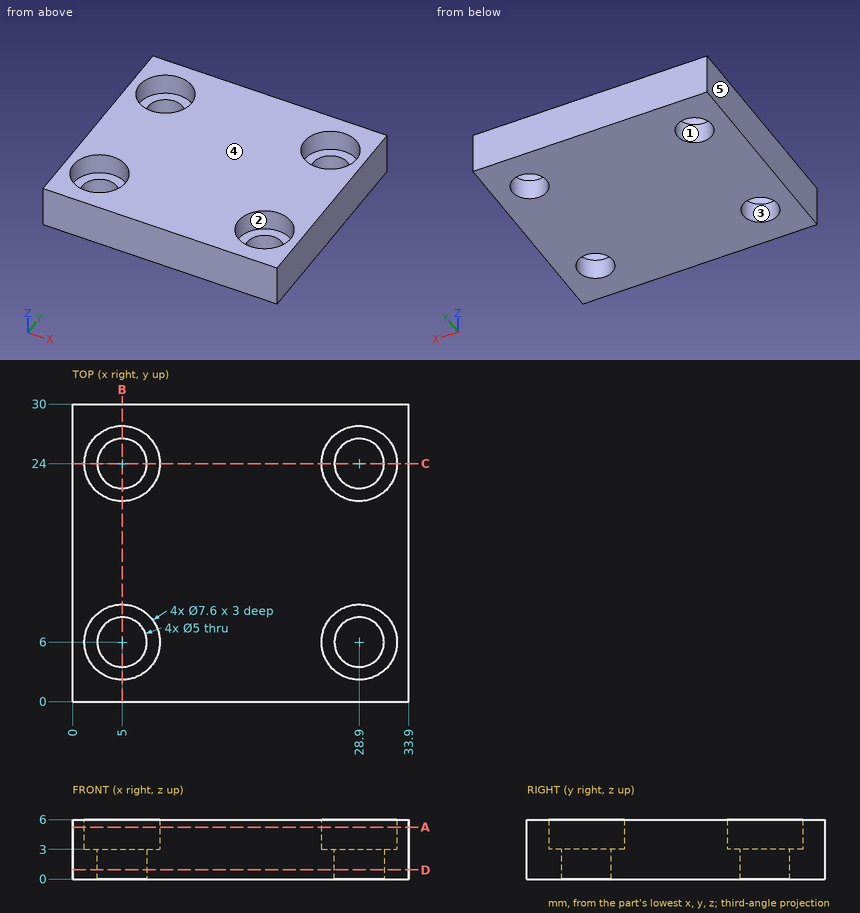
Can you work these out from the drawing? Everything is in mm from the part's minimum corner. A direction names the side the tool comes from. Give positions to 0.01 mm unless a question says otherwise; leave off trailing zeros. Order: outer loops, then holes, each group sorted by start corner. A loop starts at its lowest first (then second) coordinate and runs counter-clockwise, first axis right, second up. Notation, with made-up numbers: M 51.5,44.5 L 58.5,44.5 A24 cw 58.5,81.5 Z; hole C -22,44.25 d5. An arc over 180 degrees is marked long. Write item = value, one per line. Start each with the question number.
Q1. Suppose I cut it at A-A (z = 5.25). Write out the boundary of the cut face in (x, y), plus the area to 3 significant figures.
Q2. Suppose I cut it at C-C (y = 24). Write out the boundary of the cut face in (x, z).
Q3. For the marked faces 1 and 2, which set-ups out of +Z, -Z, +X, -X, +Y, -Y let a thin tool reach every point of the face, with its end or its side?
Q4. Will these pins go through, and if not, where does the flat tip stop? pin 1 Ø7 at (x, y) = (28.9, 6) entering from +Z; pin 2 Ø2 at (y, z) = (12, 1.5) entering from -X; pin 3 Ø2.5 at (x, y) = (6, 6) entering from +Z.
Q5. We'd pull the mould along X, two halves only. Please class the marked faces 3, 4 and 5: pulls with the +X half, pulls with the -X half, needs draft (parallel to the pull), parting line crosses it, or undercut.
Q6. I need wall thicknesses on probe 1 along Y at (x, z) = (28.9, 0.8); probe 2 along Y at (x, z) = (5, 3.3); probe 3 along X at (y, z) = (4.5, 5.15). Which ranges of each line are inside material? Lowest first, please. Write a range as [from, to].
Q7. Suppose I cut it at D-D (z = 0.95). Write out the boundary of the cut face in (x, y), plus the area to 3 significant figures.
Q8. Suppose I cut it at B-B (x = 5). Write out the boundary of the cut face in (y, z).
Check result:
q1.outline = M 0,0 L 33.9,0 L 33.9,30 L 0,30 Z; hole C 5,6 d7.6; hole C 5,24 d7.6; hole C 28.9,6 d7.6; hole C 28.9,24 d7.6
q1.area = 836 mm2
q2.outline = M 0,0 L 2.5,0 L 2.5,3 L 1.2,3 L 1.2,6 L 0,6 Z; M 7.5,0 L 26.4,0 L 26.4,3 L 25.1,3 L 25.1,6 L 8.8,6 L 8.8,3 L 7.5,3 Z; M 31.4,0 L 33.9,0 L 33.9,6 L 32.7,6 L 32.7,3 L 31.4,3 Z
q3.face_1 = +Z, -Z
q3.face_2 = +Z
q4.pin_1 = 3
q4.pin_2 = 0
q4.pin_3 = through
q5.face_3 = undercut
q5.face_4 = needs draft
q5.face_5 = pulls with the -X half
q6.probe_1 = [0, 3.5], [8.5, 21.5], [26.5, 30]
q6.probe_2 = [0, 2.2], [9.8, 20.2], [27.8, 30]
q6.probe_3 = [0, 1.51], [8.49, 25.41], [32.39, 33.9]
q7.outline = M 0,0 L 33.9,0 L 33.9,30 L 0,30 Z; hole C 5,6 d5; hole C 5,24 d5; hole C 28.9,6 d5; hole C 28.9,24 d5
q7.area = 938 mm2
q8.outline = M 0,0 L 3.5,0 L 3.5,3 L 2.2,3 L 2.2,6 L 0,6 Z; M 8.5,0 L 21.5,0 L 21.5,3 L 20.2,3 L 20.2,6 L 9.8,6 L 9.8,3 L 8.5,3 Z; M 26.5,0 L 30,0 L 30,6 L 27.8,6 L 27.8,3 L 26.5,3 Z
